Autodesk Inventor part; units mm, degrees
ref_plane "YZ Plane" through (0, 0, 0) normal (1, 0, 0) x (0, 1, 0)
ref_plane "XZ Plane" through (0, 0, 0) normal (0, 1, 0) x (-1, 0, 0)
ref_plane "XY Plane" through (0, 0, 0) normal (0, 0, 1) x (1, 0, 0)
sketch "Sketch1" plane through (0, 0, 0) normal (0, 0, 1) x (1, 0, 0)
  line L0 (-45, 45) -> (-45, -45)
  line L1 (-45, -45) -> (-25, -45)
  line L2 (-25, -45) -> (45, 25)
  line L3 (45, 25) -> (45, 45)
  line L4 (45, 45) -> (-45, 45)
  point P0 (0, 0)
  point P1 (0, 45)
  point P2 (-45, 0)
  dimension "d0" = 20
  dimension "d1" = 20
  dimension "d2" = 90
  dimension "d3" = 90
extrude "Extrusion1" add sketch "Sketch1" along normal blind 5
sketch "Sketch2" plane through (0, 0, 5) normal (0, 0, 1) x (1, 0, 0)
  circle A0 centre (-11, 11) radius 2.5
  circle A1 centre (2, -2) radius 2.5
  line L0 (-25, -45) -> (45, 25)
  line L1 (45, 45) -> (-45, 45)
  line L2 (10, -10) -> (-45, 45) construction
  line L3 (-45, 45) -> (-45, -45)
  point P0 (0, 0)
  dimension "d6" = 5
  dimension "d7" = 34
  dimension "d8" = 13
extrude "Extrusion2" cut sketch "Sketch2" against normal blind 6
ref_plane "Work Plane2" through (-11, 11, 5) normal (0.7071, -0.7071, 0) x (0.7071, 0.7071, 0)
ref_plane "Work Plane1" through (-9.2322, 9.2322, 5) normal (0.7071, -0.7071, 0) x (0.7071, 0.7071, 0)
sketch "Sketch3" plane through (-11, 11, 5) normal (0.7071, -0.7071, 0) x (0.7071, 0.7071, 0)
  line L0 (-49.4975, 0) -> (49.4975, 0)
  line L1 (0, 2) -> (0, 0)
  line L2 (-9, 0) -> (0, 0)
  line L3 (-9, 0) -> (-4, 2)
  line L4 (-4, 2) -> (0, 2)
  point P0 (0, -5)
  dimension "d12" = 9
  dimension "d13" = 2
  dimension "d17" = 4
revolve "Revolution1" add sketch "Sketch3" angle 360 about axis through (-11, 11, 7) along (0, 0, -1)
sketch "Sketch4" plane through (-11, 11, 5) normal (0, 0, -1) x (-1, 0, 0)
  circle A0 centre (0, 0) radius 2.5
  point P0 (-11, -11)
extrude "Extrusion3" cut sketch "Sketch4" against normal up to next
sketch "Sketch5" plane through (0, 0, 5) normal (0, 0, 1) x (1, 0, 0)
  circle A0 centre (-35, -37) radius 2.1
  circle A1 centre (-35, -18) radius 2.1
  circle A2 centre (-35, 20) radius 2.1
  circle A3 centre (-20, 35) radius 2.1
  circle A4 centre (-1, 35) radius 2.1
  circle A5 centre (18, 35) radius 2.1
  circle A6 centre (37, 35) radius 2.1
  line L0 (-45, -45) -> (-25, -45)
  line L1 (45, 25) -> (45, 45)
  circle A7 centre (-35, 1) radius 2.1
  point P0 (0, 0)
  point P1 (45, 35)
  point P2 (-35, -45)
  point P3 (-35, -45)
  point P4 (-35, -45)
  dimension "d18" = 4.2
  dimension "d19" = 8
  dimension "d20" = 19
  dimension "d21" = 19
  dimension "d22" = 19
  dimension "d23" = 8
  dimension "d24" = 19
  dimension "d25" = 19
  dimension "d26" = 19
extrude "Extrusion4" cut sketch "Sketch5" against normal up to next
sketch "Sketch7" plane through (0, 0, 0) normal (0, 0, -1) x (-1, 0, 0)
  line L0 (15.15, 13.396) -> (15.15, 8.604)
  line L1 (15.15, 8.604) -> (11, 6.208)
  line L2 (11, 6.208) -> (6.85, 8.604)
  line L3 (6.85, 8.604) -> (6.85, 13.396)
  line L4 (6.85, 13.396) -> (11, 15.792)
  line L5 (11, 15.792) -> (15.15, 13.396)
  circle A0 centre (11, 11) radius 2.5
  circle A1 centre (11, 11) radius 4.15 construction
  point P0 (0, 0)
  point P1 (15.15, 11)
  dimension "d30" = 8.3
  dimension "d32" = 8.3
extrude "Extrusion5" cut sketch "Sketch7" against normal blind 5
ref_plane "Work Plane4" through (2, -2, 5) normal (0.7071, -0.7071, 0) x (0.7071, 0.7071, 0)
ref_plane "Work Plane3" through (0.2322, -0.2322, 5) normal (0.7071, -0.7071, 0) x (0.7071, 0.7071, 0)
sketch "Sketch8" plane through (2, -2, 5) normal (0.7071, -0.7071, 0) x (0.7071, 0.7071, 0)
  line L0 (2.5, -5) -> (-2.5, -5)
  line L1 (-2.5, 0) -> (2.5, 0)
  line L2 (-2.5, 0) -> (2.5, 0)
  line L3 (-2.5, 0) -> (-6.5, 0)
  line L4 (-6.5, 0) -> (-4, 11.5)
  line L5 (-4, 11.5) -> (-2.5, 11.5)
  line L6 (-2.5, 0) -> (-2.5, 11.5)
  line L7 (0, 0) -> (0, 4.1579) construction
  point P0 (0, -5)
  dimension "d36" = 4
  dimension "d37" = 1.5
  dimension "d38" = 11.5
revolve "Revolution2" add sketch "Sketch8" angle 360 about axis through (2, -2, 5) along (0, 0, 1)
fillet "Fillet2" radius 2 1 edges at (6.5962, 2.5962, 5)
fillet "Fillet3" radius 2 5 edges at (-45, -45, 2.5) (-25, -45, 2.5) (45, 25, 2.5) (45, 45, 2.5) (-45, 45, 2.5)
sketch "Sketch9" plane through (0, 0, 5) normal (0, 0, 1) x (1, 0, 0)
  line L0 (45, 60.6981) -> (13, 60.6981)
  line L1 (13, 60.6981) -> (13, -8.5167)
  line L2 (13, -8.5167) -> (45, -8.5167)
  line L3 (45, -8.5167) -> (45, 60.6981)
  point P0 (0, 0)
  point P1 (45, 43)
  dimension "d42" = 32
extrude "Extrusion6" cut sketch "Sketch9" against normal up to next
equation "\"d21\" = d20"
equation "\"d22\" = d20"
equation "\"d24\" = d20"
equation "\"d25\" = d20"
equation "\"d26\" = d20"
properties part number "bracket-GT2-right"
Check sheet for the modelled part. Datum: model origin and axes. Units: mm. A direction names the side the tool comes from. Give positions to 0.01 mm unless a question says otherwise; leave off trailing zeros. Order: outer loops, then holes, each group sorted by start corner. A loop starts at its lowest first (then second) coordinate and runs counter-clockwise, first axis right, second up. Notation, with made-up numbers: M 2.5,-35 L 42.5,-35 A25 cw 42.5,-4 Z; hole C 47.5,21.5 d11. An arc over 180 degrees is marked long. Answer as CSV lines item,"result". Start each with the question number.
Item 1: Cross-section at D-D on y = 11. Enter the section's corners in (x, z), plus the area to 4 significant figures.
Item 2: Cross-section at B-B on x = -35. Enter the section's corners in (y, z), plus the area to 3 significant figures.
Item 3: Gauge pin test, flat ends, axial feed: P1, Ø4, axis at x = -9.5, y = 10.5, coming from the -Z side; P2, Ø5.5, axis at x = -20, y = 35, coming from the +Z side; P3, Ø3.5, axis at x = -1, y = 35, coming from the -Z side; P4, Ø17.5, axis at x = -11.5, y = 8.5, coming from the +Z side. Record the tip position at first contact, or that the pin passes through.
Item 4: Mould release check, pull along X, two halves, no side actions. Record for faces 1 (the face through (-45, 1, 2)), 2 (the face through (-36.548, -16.581, 2.535)), 3 (the face through (-16, 1, 0)): +X half, -X half, draft (parallel to the pull), parting line (faces both ways), or undercut.
Item 5: Cross-section at C-C on x = 2. Enter the section's corners in (y, z).
Item 6: Thickness scan on line 1 (Y direction, x = -35, z = 3.35); line 2 (Y direction, x = -36, z = 4.5); line 3 (Z direction, x = -1.5, y = 17.5). Record the ranges inside material, lowest first. Write a range as [from, to].
Item 7: Cross-section at A-A on y = -18. Enter the section's corners in (x, z), plus the area to 3 significant figures.
Item 8: Tool access check on faces 4 (the face through (-9, 9, 5)), 5 (the face through (-36.666, -38.278, 2.535)). Record the directions out of +Z, -Z, +X, -X, +Y, -Y that give a thin tool (end or side, any length) a straight path to the whole face; none if there is none.
Established:
1,outline,"M -45,0 L -15.15,0 L -15.15,5 L -13.5,5 L -13.5,7 L -15,7 L -20,5 L -45,5 Z; M -8.5,5 L -6.85,5 L -6.85,0 L 13,0 L 13,5 L -2,5 L -7,7 L -8.5,7 Z"
1,area,"264.5 mm^2"
2,outline,"M -45,0 L -39.1,0 L -39.1,5 L -45,5 Z; M -34.9,0 L -20.1,0 L -20.1,5 L -34.9,5 Z; M -15.9,0 L -1.1,0 L -1.1,5 L -15.9,5 Z; M 3.1,0 L 17.9,0 L 17.9,5 L 3.1,5 Z; M 22.1,0 L 45,0 L 45,5 L 22.1,5 Z"
2,area,"366 mm^2"
3,P1,"stops at z = 5"
3,P2,"stops at z = 5"
3,P3,"passes through"
3,P4,"stops at z = 7"
4,face 1,"-X half"
4,face 2,"undercut"
4,face 3,"draft"
5,outline,"M -18,0 L -4.5,0 L -4.5,16.5 L -6,16.5 L -8.16,6.58 A2 cw -10.11,5 L -18,5 Z; M 0.5,0 L 45,0 L 45,5 L 6.11,5 A2 cw 4.16,6.58 L 2,16.5 L 0.5,16.5 Z"
6,line 1,"y = [-45, -39.1], [-34.9, -20.1], [-15.9, -1.1], [3.1, 17.9], [22.1, 45]"
6,line 2,"y = [-45, -38.85], [-35.15, -19.85], [-16.15, -0.85], [2.85, 18.15], [21.85, 45]"
6,line 3,"z = [0, 5]"
7,outline,"M -45,0 L -37.1,0 L -37.1,5 L -45,5 Z; M -32.9,0 L 2,0 L 2,5 L -32.9,5 Z"
7,area,"214 mm^2"
8,face 4,"-Z"
8,face 5,"+Z, -Z"
